Geometry: final body of the model. Coordinates: model frame, mm. A direction names the side the tool comes from. Give positions to 0.01 mm unless a question says otherwise; leave off trailing zeros. Order: outer loops, then holes, each group sorted by start corner. A loop starts at its lowest first (then second) coordinate and runs counter-clockwise, first axis right, second up. Notation, with made-up numbers: (77.25, -24.75) -> (127.25, -24.75) arc R22 cw to (127.25, -8.75) -> close; hole circle Ø11 at (-4.75, 60.5). An arc over 180 degrees is marked (long way). Answer in a Markdown table with one row per item. Add a question column.
Q1. Line query: line 1 along X through (y, z) = (12, 9.5); line 2 along X through (y, z) = (11.5, 7.5); line 3 along Y through (x, z) = (-71.5, 6.25). Output: solid intervals per line, ascending. Write a range as from..to.
Q2. Cut plane A-A on x = 35. Return the cut outline in (y, z).
Q3. Set-up query: faces 1 (the face through (-84.35, 26, 9)), 2 (the face through (35, 16.472, 9)), 3 (the face through (41.65, 25, 9)), 4 (the face through (-22, 13, 0)), 5 (the face through (-76, 20.472, 9)). Return all of +Z, -Z, +X, -X, +Y, -Y with unobstructed straight access to the full face (end or side cutting, diameter ignored); none if empty.
Q4. Pull-direction query (X, two-part tool) for faces 6 (the face through (-77, 16.472, 9)), 7 (the face through (-86.35, 6, 9)), 8 (the face through (10.513, 14.091, 8.874)); classes: +X half, -X half, draft (parallel to the pull), parting line (faces both ways), or undercut.
Q5. Cut plane C-C on y = 10.5. Return the cut outline in (x, z).
Q6. Contact query for a flat-ended pin moving along its axis: P1, Ø1, axis at y = 19, z = 8, coming from the -X side. Output: stop coordinate, or through.
Q7. Cut plane D-D on x = 16. Return the cut outline in (y, z).
Q8. Cut plane B-B on z = 12.5. Return the cut outline in (x, y), and give its area (3 significant figures).
from build123d import *

# Parameters (mm, degrees)
F0_R     = 13
F1_DEPTH = 18
F2_DEPTH = 2
F3_DEPTH = 2


with BuildPart() as f1:
    # F0 (on Top) → F1 (new body)
    with BuildSketch(Plane.XY):
        with BuildLine():
            Line((43.6501808017, 30.4717739075), (-86.3498191983, 30.4717739075))
            Line((-86.3498191983, 30.4717739075), (-86.3498191983, 20.4717739075))
            Line((-86.3498191983, 20.4717739075), (-67.7780224285, 20.4717739075))
            ThreePointArc((-67.7780224285, 20.4717739075), (-58.7792668374, 24.1991805179), (-52.8498191983, 16.4717739075))
            ThreePointArc((-52.8498191983, 16.4717739075), (-60.8498191983, 8.4717739075), (-68.8498191983, 16.4717739075))
            Line((-68.8498191983, 16.4717739075), (-86.3498191983, 16.4717739075))
            Line((-86.3498191983, 16.4717739075), (-86.3498191983, -5.5282260925))
            Line((-86.3498191983, -5.5282260925), (43.6501808017, -5.5282260925))
            Line((43.6501808017, -5.5282260925), (43.6501808017, 16.4717739075))
            Line((43.6501808017, 16.4717739075), (26.1501808017, 16.4717739075))
            ThreePointArc((26.1501808017, 16.4717739075), (10.4227741914, 14.4012215467), (25.078384032, 20.4717739075))
            Line((25.078384032, 20.4717739075), (43.6501808017, 20.4717739075))
            Line((43.6501808017, 20.4717739075), (43.6501808017, 30.4717739075))
        make_face()
        with Locations((-21.3498191983, 16.4717739075)):
            Circle(F0_R, mode=Mode.SUBTRACT)
        with Locations((-21.3498191983, 16.4717739075)):
            Circle(F0_R)
    extrude(amount=F1_DEPTH)

    # F2 (cut): a face of the model
    f2_faces = [f1.faces().sort_by_distance(p)[0] for p in [
        (-86.3498191983, 25.4717739075, 9),
    ]]
    extrude(f2_faces, amount=-F2_DEPTH, mode=Mode.SUBTRACT)

    # F3 (cut): a face of the model
    f3_faces = [f1.faces().sort_by_distance(p)[0] for p in [
        (43.6501808017, 25.4717739075, 9),
    ]]
    extrude(f3_faces, amount=-F3_DEPTH, mode=Mode.SUBTRACT)


solid = f1.part
Completed:
| question | item | result |
|---|---|---|
| 1 | line 1 | x = -86.35..-67.48, -54.22..11.52, 24.78..43.65 |
| 1 | line 2 | x = -86.35..-67.12, -54.58..11.88, 24.42..43.65 |
| 1 | line 3 | y = -5.53..16.47, 20.47..30.47 |
| 2 | outline | (-5.53, 0) -> (16.47, 0) -> (16.47, 18) -> (-5.53, 18) -> close; (20.47, 0) -> (30.47, 0) -> (30.47, 18) -> (20.47, 18) -> close |
| 3 | face 1 | +Z, -Z, -X, +Y |
| 3 | face 2 | +Z, -Z, +X |
| 3 | face 3 | +Z, -Z, +X, +Y |
| 3 | face 4 | -Z, +X, -X, +Y, -Y |
| 3 | face 5 | +Z, -Z, -X |
| 4 | face 6 | draft |
| 4 | face 7 | -X half |
| 4 | face 8 | undercut |
| 5 | outline | (-86.35, 0) -> (-66.17, 0) -> (-66.17, 18) -> (-86.35, 18) -> close; (-55.53, 0) -> (12.83, 0) -> (12.83, 18) -> (-55.53, 18) -> close; (23.47, 0) -> (43.65, 0) -> (43.65, 18) -> (23.47, 18) -> close |
| 6 | P1 | stops at x = -53.45 |
| 7 | outline | (-5.53, 0) -> (8.77, 0) -> (8.77, 18) -> (-5.53, 18) -> close; (24.18, 0) -> (30.47, 0) -> (30.47, 18) -> (24.18, 18) -> close |
| 8 | outline | (-86.35, -5.53) -> (43.65, -5.53) -> (43.65, 16.47) -> (26.15, 16.47) arc R8 cw (long way) to (25.08, 20.47) -> (41.65, 20.47) -> (41.65, 30.47) -> (-84.35, 30.47) -> (-84.35, 20.47) -> (-67.78, 20.47) arc R8 cw (long way) to (-68.85, 16.47) -> (-86.35, 16.47) -> close |
| 8 | area | 4,100 mm² |
